Could you check a few things on this model? Use its own coordinates, in mm. Face numbers are marked on the shaded views. A direction names the side the tool comes from. Round coordinates to 2 decimals unless told otherwise and drop trailing zeros. Order: outer loops, then holes, each group sorted by start corner. A loop starts at its lowest first (then second) coordinate and runs counter-clockwise, first axis right, second up. Notation, with made-up numbers: (-21, 74.25) - (17, 74.25) arc R23 cw to (17, 83.25) - close; hole circle Ø8 at (-17.5, 66.5). An arc over 180 degrees is marked (long way). Use one line per item in the form item = value.
from build123d import *

# Parameters (mm, degrees)
BOSS_EXTRUDE1_DEPTH = 25.4
SKETCH3_W           = 125.222
SKETCH3_H           = 152.4
BOSS_EXTRUDE2_DEPTH = 2.54
SKETCH5_W           = 38.1
SKETCH5_H           = 152.4
CUT_EXTRUDE1_DEPTH  = 1.27


with BuildPart() as part:
    # Sketch1 → Boss-Extrude1 (new body)
    with BuildSketch(Plane(origin=(0, 0, 0), x_dir=(1, 0, 0), z_dir=(0, 1, 0))):
        Polygon((-64.654545455, 257.896590909), (-39.254545455, 257.896590909), (-39.254545455, -21.503409091), (35.167454545, -21.503409091), (35.167454545, 257.896590909), (60.567454545, 257.896590909), (60.567454545, -46.903409091), (-64.654545455, -46.903409091), align=None)
    extrude(amount=BOSS_EXTRUDE1_DEPTH)

    # Sketch3 → Boss-Extrude2 (add)
    with BuildSketch(Plane(origin=(0, 25.4, 0), x_dir=(1, 0, 0), z_dir=(0, 1, 0))):
        with Locations((-2.043545455, 29.287074317)):
            Rectangle(SKETCH3_W, SKETCH3_H)
    extrude(amount=BOSS_EXTRUDE2_DEPTH)

    # Sketch5 → Cut-Extrude1 (cut)
    with BuildSketch(Plane(origin=(0, 27.94, 0), x_dir=(1, 0, 0), z_dir=(0, 1, 0))):
        with Locations((-2.043545455, 30.25907177)):
            Rectangle(SKETCH5_W, SKETCH5_H)
    extrude(amount=-CUT_EXTRUDE1_DEPTH, mode=Mode.SUBTRACT)


solid = part.part
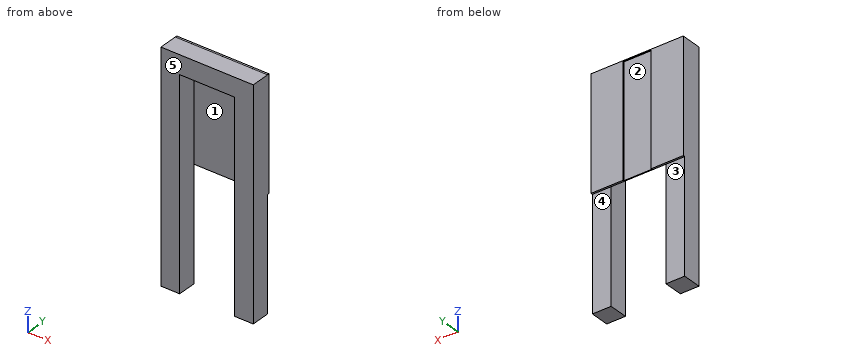
Item 1: If we mould it in two halves opening along X, with no side actions, what happens to the marked faces 1, 2 and 3? For each: released by +X, released by -X, zero draft, split by the parting line, or undercut.
Found:
face_1 = undercut
face_2 = undercut
face_3 = zero draft
Item 2: Will these pins go through, and if not, where does the flat tip stop? P1, Ø7.5, axis at x = -13.5, y = 16, coming from the -Z side; P2, Ø0.8, axis at x = -7.5, y = 26.5, coming from the -Z side; P3, Ø12.5, axis at x = 42.5, z = -161, coming from the +Y side.
Found:
P1 = 21.5
P2 = -105.49
P3 = 25.4
Item 3: Imagine slicing it at A-A on z = -134. Please give me the cut outline in (x, y), plus the area to 3 significant figures.
Found:
outline = (-64.65, 0) - (-39.25, 0) - (-39.25, 25.4) - (-64.65, 25.4) - close; (35.17, 0) - (60.57, 0) - (60.57, 25.4) - (35.17, 25.4) - close
area = 1,290 mm2
Item 4: For the marked faces 4 and 5, which set-ups out of +Z, -Z, +X, -X, +Y, -Y let a thin tool reach every point of the face, with its end or its side?
Found:
face_4 = -Z, +X, -X, +Y
face_5 = +Z, -Z, +X, -X, -Y
Item 5: Imagine slicing it at C-C on y = 11.5. Please give me the cut outline in (x, z), plus the area to 3 significant figures.
Found:
outline = (-64.65, -257.9) - (-39.25, -257.9) - (-39.25, 21.5) - (35.17, 21.5) - (35.17, -257.9) - (60.57, -257.9) - (60.57, 46.9) - (-64.65, 46.9) - close
area = 17,400 mm2
Item 6: I need wall thicknesses on L1, parallel to X at y = 4, z = -190.5; L2, parallel to Z at x = -16.5, y = 21; L3, parallel to Y at x = -6, z = -85. Which ranges of each line are inside material? Lowest first, please.
Found:
L1 = -64.65 to -39.25, 35.17 to 60.57
L2 = 21.5 to 46.9
L3 = 25.4 to 26.67
Item 7: Imagine slicing it at D-D on z = -38.5. Please give me the cut outline in (x, y).
Found:
outline = (-64.65, 0) - (-39.25, 0) - (-39.25, 25.4) - (35.17, 25.4) - (35.17, 0) - (60.57, 0) - (60.57, 27.94) - (17.01, 27.94) - (17.01, 26.67) - (-21.09, 26.67) - (-21.09, 27.94) - (-64.65, 27.94) - close
